```python
from build123d import *

# Parameters (mm, degrees)
SKETCH1_R           = 7.5
BOSS_EXTRUDE1_DEPTH = 58
SKETCH2_W           = 38
SKETCH2_H           = 30
SKETCH2_W_2         = 16
SKETCH2_H_2         = 42
CUT_EXTRUDE1_DEPTH  = 58
CUT_EXTRUDE2_DEPTH  = 58
SKETCH4_R           = 7
CUT_EXTRUDE3_DEPTH  = 108
CUT_EXTRUDE4_DEPTH  = 6
CUT_EXTRUDE5_DEPTH  = 12


with BuildPart() as part:
    # Sketch1 → Boss-Extrude1 (new body)
    with BuildSketch(Plane(origin=(0, 0, 0), x_dir=(1, 0, 0), z_dir=(0, 1, 0))):
        with BuildLine():
            Line((0, 0), (65, 0))
            Line((65, 0), (80, 8.660254038))
            Line((80, 8.660254038), (80, 31.339745962))
            Line((80, 31.339745962), (65, 40))
            Line((65, 40), (36.66060556, 40))
            ThreePointArc((36.66060556, 40), (16.66060556, 35.82575695), (0, 24))
            Line((0, 24), (0, 0))
        make_face()
        with Locations(Location((34, 19, 0), (0, 0, 90))):
            Circle(SKETCH1_R, mode=Mode.SUBTRACT)
    extrude(amount=BOSS_EXTRUDE1_DEPTH)

    # Sketch2 → Cut-Extrude1 (cut)
    with BuildSketch(Plane.XY):
        with Locations((35, 29)):
            Rectangle(SKETCH2_W, SKETCH2_H)
        with Locations((8, 29)):
            Rectangle(SKETCH2_W_2, SKETCH2_H_2)
    extrude(amount=-CUT_EXTRUDE1_DEPTH, mode=Mode.SUBTRACT)

    # Sketch3 → Cut-Extrude2 (cut)
    with BuildSketch(Plane.XY):
        Polygon((65, 58), (80, 58), (80, 43), align=None)
        Polygon((65, 0), (80, 0), (80, 15), align=None)
    extrude(amount=-CUT_EXTRUDE2_DEPTH, mode=Mode.SUBTRACT)

    # Sketch4 → Cut-Extrude3 (cut)
    with BuildSketch(Plane(origin=(0, 0, 0), x_dir=(0, 0, -1), z_dir=(1, 0, 0))):
        with Locations(Location((20, 29, 0), (0, 0, 180))):
            Circle(SKETCH4_R)
    extrude(amount=CUT_EXTRUDE3_DEPTH, mode=Mode.SUBTRACT)

    # Sketch5 → Cut-Extrude4 (cut)
    with BuildSketch(Plane(origin=(0, 0, 0), x_dir=(1, 0, 0), z_dir=(0, 1, 0))):
        with BuildLine():
            Line((0, 20.98386677), (0, 2))
            Line((0, 2), (63, 2))
            Line((63, 2), (63, 38))
            Line((63, 38), (36.66060556, 38))
            ThreePointArc((36.66060556, 38), (16.452013389, 33.538635744), (0, 20.98386677))
        make_face()
    extrude(amount=CUT_EXTRUDE4_DEPTH, mode=Mode.SUBTRACT)

    # Sketch7 → Cut-Extrude5 (cut)
    with BuildSketch(Plane(origin=(0, 0, 0), x_dir=(1, 0, 0), z_dir=(0, 1, 0))):
        with BuildLine():
            Line((18, 32.044997326), (18, 4))
            Line((18, 4), (61, 4))
            Line((61, 4), (61, 36))
            Line((61, 36), (36.66060556, 36))
            ThreePointArc((36.66060556, 36), (27.123044996, 35.000388204), (18, 32.044997326))
        make_face()
    extrude(amount=CUT_EXTRUDE5_DEPTH, mode=Mode.SUBTRACT)


solid = part.part
```
Geometry check sheet. Reference: the model listing, model coordinates, mm. A direction names the side the tool comes from. Round coordinates to 2 decimals unless told otherwise and drop trailing zeros. Loops run counter-clockwise (first coordinate to the right, second up) from the corner with the lowest first, then second, coordinate; pieces in that order, holes last. Notation, with made-up numbers: (70.5, 10.5) - (98.5, 10.5) arc R29 ccw to (98.5, 39.5) - close; hole circle Ø5 at (56, -20.5). An arc over 180 degrees is marked (long way). Write each question's results on one line, items separated by ' | '. Start each with the question number.
Q1. Cross-section at B-B on x = 48.5. Enter the section's corners in (y, z).
Q2. Cross-section at D-D on x = 60. Enter the section's corners in (y, z), and give its area (3 significant figures).
Q3. Cross-section at C-C on z = -14.5. State how many separate pieces and enclosed holes the cut face has, and give its area (3 significant figures).
Q4. Release check for a two-part mould opening along Z. For faces 1 (the flat face through (39, 9, 0)), 2 (the flat face through (63, 3, -20)), 3 (the flat face through (8, 8, -14)) record: +Z half, -Z half, draft (parallel to the pull), parting line (faces both ways), or undercut.
Q5. Cross-section at A-A on y = 29. Enter the section's corners in (x, z).
Q6. Gauge pin test, flat ends, axial feed: P1, Ø6, axis at x = 59, z = -15.5, coming from the -Y side; P2, Ø4, axis at y = 25, z = -29, coming from the -X side; P3, Ø5, axis at x = 54.5, y = 1.5, coming from the +Z side; P4, Ø19, axis at x = 41.5, z = -17.5, coming from the -Y side. Record the tip position at first contact, or that the pin passes through.
Q7. Access from +Z, -Z, +X, -X, +Y, -Y to the whole of each face (thin tool, end or side, straight path). Record for faces 4 (the flat face through (17, 6, -16)), 5 (the flat face through (43, 44, -20)), 6 (the flat face through (31, 3, -2)).
Q8. Thickness scan on line 1 (Y direction, x = 23, z = -29); line 2 (Z direction, x = 50, y = 7); line 3 (Y direction, x = 10, z = -14). Record the ranges inside material, lowest first. Write a range as [from, to].
Answers below:
1) outline: (0, -40) - (14, -40) - (14, 0) - (0, 0) - (0, -2) - (6, -2) - (6, -4) - (12, -4) - (12, -36) - (6, -36) - (6, -38) - (0, -38) - close; (44, -40) - (58, -40) - (58, 0) - (44, 0) - close
2) outline: (0, -40) - (58, -40) - (58, 0) - (0, 0) - (0, -2) - (6, -2) - (6, -4) - (12, -4) - (12, -36) - (6, -36) - (6, -38) - (0, -38) - close; hole circle Ø14 at (29, -20) | area: 1,760 mm²
3) separate pieces: 4 | enclosed holes: 0 | area: 1,550 mm²
4) face 1: +Z half | face 2: undercut | face 3: draft
5) outline: (54, -40) - (65, -40) - (80, -31.34) - (80, -27) - (54, -27) - close; (54, -13) - (80, -13) - (80, -8.66) - (65, 0) - (54, 0) - close
6) P1: stops at y = 6 | P2: stops at x = 54 | P3: stops at z = 0 | P4: stops at y = 12
7) face 4: -Y | face 5: +Z, -Z, -X | face 6: -X, -Y
8) line 1: y = [12, 14], [44, 58] | line 2: z = [-40, -36], [-4, 0] | line 3: y = [6, 8], [50, 58]
